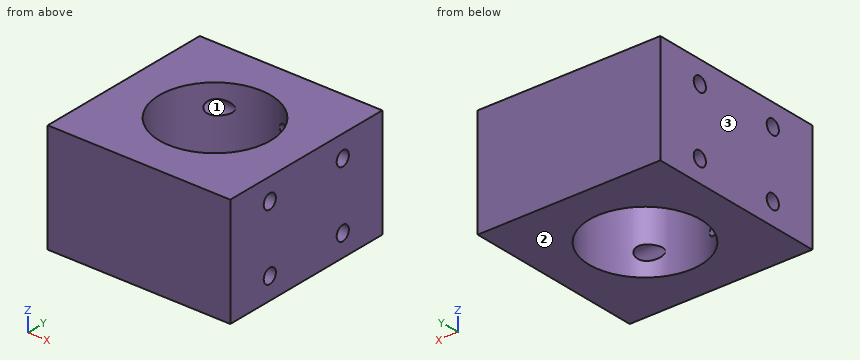
```python
from build123d import *

# Parameters (mm, degrees)
F0_W     = 50
F0_H     = 30
F0_R     = 2
F1_DEPTH = 25
F2_R     = 15.25
F3_DEPTH = 30.001


# Not quite as in the source:
# - a feature names something its author has since deleted; it is built from what else it names


with BuildPart() as f1:
    # F0 (on Right) → F1 (new body, symmetric)
    with BuildSketch(Plane.YZ):
        Rectangle(F0_W, F0_H)
        with Locations((-12.0000001043, -9)):
            Circle(F0_R, mode=Mode.SUBTRACT)
        with Locations((12.0000001043, -9)):
            Circle(F0_R, mode=Mode.SUBTRACT)
        with Locations((-12, 9)):
            Circle(F0_R, mode=Mode.SUBTRACT)
        with Locations((12, 9)):
            Circle(F0_R, mode=Mode.SUBTRACT)
    extrude(amount=F1_DEPTH, both=True)

    # F2 (on face) → F3 (cut, through all)
    with BuildSketch(Plane.XY.offset(15)):
        Circle(F2_R)
    extrude(amount=-F3_DEPTH, mode=Mode.SUBTRACT)


solid = f1.part
```
For this review, take the finished solid that the model builds, in its own axes (mm). Face numbers are marked on the shaded views. Round coordinates to 2 decimals unless told otherwise and drop trailing zeros. Write each loop counter-clockwise with the first axis right and the second up, starting at its lowest first coordinate (ties: lowest second). Pieces come first, ordered by that corner, then holes. Notation, with made-up numbers: M 0,3.5 L 17,3.5 A21 ccw 17,32.5 Z; hole C 19,-38.75 d10. An arc over 180 degrees is marked long. One line per item, written item: value. Start each with the question number.
(1) We need section D-D (x = 10). Give the boundary of the cut face in (y, z).
(2) The part is to be moulded in two halves that separate along Z. For the marked faces 1, 2 and 3, say which applies: released by +Z, released by -Z, zero draft, split by the parting line, or undercut.
(3) We need section B-B (x = -22). Give the boundary of the cut face in (y, z).
(4) We need section C-C (z = -9). Give the boundary of the cut face in (x, y).
(5) Wall thickness on line 1 (Z direction, x = -18, y = -12); line 2 (Y direction, x = 19.75, z = 9); line 3 (Y direction, x = 12, z = -9): over which ranges is each line inside the solid? List them lowest first.
(6) We need section A-A (y = -11). Give the boundary of the cut face in (x, z).
Result:
1. outline: M -25,-15 L -11.51,-15 L -11.51,-10.94 A2 cw long -11.51,-7.06 L -11.51,7.06 A2 cw long -11.51,10.94 L -11.51,15 L -25,15 Z; M 11.51,-15 L 25,-15 L 25,15 L 11.51,15 L 11.51,10.94 A2 cw long 11.51,7.06 L 11.51,-7.06 A2 cw long 11.51,-10.94 Z
2. face 1: undercut
2. face 2: released by -Z
2. face 3: zero draft
3. outline: M -25,-15 L 25,-15 L 25,15 L -25,15 Z; hole C -12,-9 d4; hole C -12,9 d4; hole C 12,-9 d4; hole C 12,9 d4
4. outline: M -25,-25 L 25,-25 L 25,-14 L 6.05,-14 A15.25 cw -6.05,-14 L -25,-14 Z; M -25,-10 L -11.51,-10 A15.25 cw -11.51,10 L -25,10 Z; M -25,14 L -6.05,14 A15.25 cw 6.05,14 L 25,14 L 25,25 L -25,25 Z; M 11.51,-10 L 25,-10 L 25,10 L 11.51,10 A15.25 cw Z
5. line 1: -15 to -11, -7 to 7, 11 to 15
5. line 2: -25 to -14, -10 to 10, 14 to 25
5. line 3: -25 to -14, -10 to -9.41, 9.41 to 10, 14 to 25
6. outline: M -25,-15 L -10.56,-15 L -10.56,-10.73 L -25,-10.73 Z; M -25,-7.27 L -10.56,-7.27 L -10.56,7.27 L -25,7.27 Z; M -25,10.73 L -10.56,10.73 L -10.56,15 L -25,15 Z; M 10.56,-15 L 25,-15 L 25,-10.73 L 10.56,-10.73 Z; M 10.56,-7.27 L 25,-7.27 L 25,7.27 L 10.56,7.27 Z; M 10.56,10.73 L 25,10.73 L 25,15 L 10.56,15 Z
